```python
from build123d import *

# Parameters (mm, degrees)
BOSS_EXTRUDE1_DEPTH = 50


with BuildPart() as part:
    # Sketch1 → Boss-Extrude1 (new body)
    with BuildSketch(Plane(origin=(0, 0, 0), x_dir=(1, 0, 0), z_dir=(0, 1, 0))):
        with BuildLine():
            Line((-187.507179986, -35.023134548), (-64.632225867, -692.872194477))
            ThreePointArc((-64.632225867, -692.872194477), (0, -746.55), (64.632225867, -692.872194477))
            Line((64.632225867, -692.872194477), (187.507179986, -35.023134548))
            ThreePointArc((187.507179986, -35.023134548), (0, 190.75), (-187.507179986, -35.023134548))
        make_face()
        with BuildLine():
            ThreePointArc((-44.972233208, -689.200044066), (0, -726.55), (44.972233208, -689.200044066))
            Line((44.972233208, -689.200044066), (167.847187327, -31.350984136))
            ThreePointArc((167.847187327, -31.350984136), (0, 170.75), (-167.847187327, -31.350984136))
            Line((-167.847187327, -31.350984136), (-44.972233208, -689.200044066))
        make_face(mode=Mode.SUBTRACT)
    extrude(amount=BOSS_EXTRUDE1_DEPTH)


solid = part.part
```
Check sheet for the modelled part. Datum: model origin and axes. Units: mm. A direction names the side the tool comes from. Coordinates: 2 decimals unless noted, no trailing zeros. Write each loop counter-clockwise with the first axis right and the second up, starting at its lowest first coordinate (ties: lowest second). Pieces come first, ordered by that corner, then holes. Notation, with made-up numbers: M -24,-38 L -17,-38 A21 cw -17,-15 Z; hole C 7.25,81 d5. An arc over 180 degrees is marked long. Write item = value, one per line. Start each with the question number.
1. Sectioned sample at B-B (z = 0). Record the cut outline in (x, y), then the cut area to 3 significant figures.
2. Sectioned sample at A-A (x = 0). Record the cut outline in (y, z).
3. Go/stop test with flat-tipped pins: pin 1 (3 mm diameter, centred on y = 44.5, z = 467, fed in from +X); pin 2 (10 mm diameter, centred on y = 21, z = 406, fed in from +X); pin 3 (12 mm diameter, centred on x = 94, y = 44.5, fed in from -Z). Record where each tip stops, or that it passes through.
4. Thickness scan on probe 1 along X at (y, z) = (17, 0); probe 2 along X at (y, z) = (6.5, 23); probe 3 along Z at (x, y) = (-41, 41). Record the ranges inside material, lowest first.
5. Sectioned sample at C-C (y = 22.5). Record the cut outline in (x, z).
6. Mould release check, pull along Z, two halves, no side actions. Record for faces 3 (the flat face through (-128, 50, 276)), 4 (the flat face through (105.55, 24.65, 364.88)), 5 (the flat face through (-126.93, 24.65, 359.34)): pulls with the +Z half, pulls with the -Z half, needs draft (parallel to the pull), parting line crosses it, or undercut.
7. Tool access check on faces 1 (the cylindrical face through (-1.276, 24.65, 746.538)), 2 (the cylindrical face through (-0.89, 24.65, 726.54)). Record the directions out of +Z, -Z, +X, -X, +Y, -Y that give a thin tool (end or side, any length) a straight path to the whole face; none if there is none.
The answers:
q1.outline = M -190.75,0 L -170.75,0 L -170.75,50 L -190.75,50 Z; M 170.75,0 L 190.75,0 L 190.75,50 L 170.75,50 Z
q1.area = 2,000 mm²
q2.outline = M 0,-190.75 L 50,-190.75 L 50,-170.75 L 0,-170.75 Z; M 0,726.55 L 50,726.55 L 50,746.55 L 0,746.55 Z
q3.pin_1 = 107.1
q3.pin_2 = 119.15
q3.pin_3 = -169.24
q4.probe_1 = -190.75 to -170.75, 170.75 to 190.75
q4.probe_2 = -189.36 to -169.19, 169.19 to 189.36
q4.probe_3 = -186.29 to -165.75, 701.1 to 732.2
q5.outline = M -187.51,35.02 A190.75 ccw long 187.51,35.02 L 64.63,692.87 A65.75 ccw -64.63,692.87 Z; hole M -167.85,31.35 A170.75 ccw long 167.85,31.35 L 44.97,689.2 A45.75 ccw -44.97,689.2 Z
q6.face_3 = needs draft
q6.face_4 = undercut
q6.face_5 = pulls with the +Z half
q7.face_1 = +Z, +Y, -Y
q7.face_2 = +Y, -Y
